Model file for the job. Use its own axes, mm. A direction names the side the tool comes from. Give positions to 0.01 mm unless a question says otherwise; leave off trailing zeros.
```python
from build123d import *

# Parameters (mm, degrees)
SKETCH1_R           = 3.5
BOSS_EXTRUDE1_DEPTH = 3.25
CUT_EXTRUDE1_DEPTH  = 2.75
SKETCH3_R           = 1.5
CUT_EXTRUDE2_DEPTH  = 6.662375826
BOSS_EXTRUDE6_DEPTH = 0.5
BOSS_EXTRUDE4_START = -2
SKETCH6_W           = 3.5
SKETCH6_H           = 2.5
BOSS_EXTRUDE4_DEPTH = 2.5
SKETCH7_W           = 2
SKETCH7_H           = 1.25
CUT_EXTRUDE3_DEPTH  = 2.23
SKETCH8_R           = 0.59
CUT_EXTRUDE4_DEPTH  = 4
CHAMFER3_SIZE       = 0.5
CIRPATTERN1_COUNT   = 3
CHAMFER4_SIZE       = 0.25


# Some blends are built 0.0001 mm under size
with BuildPart() as part:
    # Sketch1 → Boss-Extrude1 (new body)
    with BuildSketch(Plane(origin=(0, 0, 0), x_dir=(1, 0, 0), z_dir=(0, 1, 0))):
        with Locations(Location((0, 0, 0), (0, 0, 90))):
            Circle(SKETCH1_R)
    extrude(amount=BOSS_EXTRUDE1_DEPTH)

    # Sketch2 → Cut-Extrude1 (cut)
    with BuildSketch(Plane(origin=(0, 3.25, 0), x_dir=(1, 0, 0), z_dir=(0, 1, 0))):
        Polygon((1.327905619, -2.3), (2.655811238, 0), (1.327905619, 2.3), (-1.327905619, 2.3), (-2.655811238, 0), (-1.327905619, -2.3), align=None)
    extrude(amount=-CUT_EXTRUDE1_DEPTH, mode=Mode.SUBTRACT)

    # Sketch3 → Cut-Extrude2 (cut, through all)
    with BuildSketch(Plane(origin=(0, 0.5, 0), x_dir=(1, 0, 0), z_dir=(0, 1, 0))):
        with Locations(Location((0, 0, 0), (0, 0, 270))):
            Circle(SKETCH3_R)
    extrude(amount=-CUT_EXTRUDE2_DEPTH, mode=Mode.SUBTRACT)

    # Sketch4 → Boss-Extrude6 (add)
    with BuildSketch(Plane.XZ):
        with BuildLine():
            Line((-1.5, 4.5), (-1.5, 3.16227766))
            ThreePointArc((-1.5, 3.16227766), (0, 3.5), (1.5, 3.16227766))
            Line((1.5, 3.16227766), (1.5, 4.5))
            Line((1.5, 4.5), (1.5, 6))
            Line((1.5, 6), (-1.5, 6))
            Line((-1.5, 6), (-1.5, 4.5))
        make_face()
        with BuildLine():
            Line((4.647114317, -0.950961894), (3.488612788, -0.282100724))
            ThreePointArc((3.488612788, -0.282100724), (3.031088913, -1.75), (1.988612788, -2.880176936))
            Line((1.988612788, -2.880176936), (3.147114317, -3.549038106))
            Line((3.147114317, -3.549038106), (4.647114317, -0.950961894))
        make_face()
        with BuildLine():
            Line((-3.147114317, -3.549038106), (-1.988612788, -2.880176936))
            ThreePointArc((-1.988612788, -2.880176936), (-3.031088913, -1.75), (-3.488612788, -0.282100724))
            Line((-3.488612788, -0.282100724), (-4.647114317, -0.950961894))
            Line((-4.647114317, -0.950961894), (-3.147114317, -3.549038106))
        make_face()
        with BuildLine():
            Line((1.5, -4.5), (1.5, -3.16227766))
            ThreePointArc((1.5, -3.16227766), (0, -3.5), (-1.5, -3.16227766))
            Line((-1.5, -3.16227766), (-1.5, -4.5))
            Line((-1.5, -4.5), (-1.5, -6))
            Line((-1.5, -6), (1.5, -6))
            Line((1.5, -6), (1.5, -4.5))
        make_face()
    extrude(amount=-BOSS_EXTRUDE6_DEPTH)

    # Sketch6 → Boss-Extrude4 (add)
    with BuildSketch(Plane.XY.offset(-2.8).offset(BOSS_EXTRUDE4_START)):
        with Locations((0, 2)):
            Rectangle(SKETCH6_W, SKETCH6_H)
    boss_extrude4 = extrude(amount=BOSS_EXTRUDE4_DEPTH)

    # Sketch7 → Cut-Extrude3 (cut)
    with BuildSketch(Plane(origin=(0, 3.25, 0), x_dir=(1, 0, 0), z_dir=(0, 1, 0))):
        with Locations((0, 3.425)):
            Rectangle(SKETCH7_W, SKETCH7_H)
    cut_extrude3 = extrude(amount=-CUT_EXTRUDE3_DEPTH, mode=Mode.SUBTRACT)

    # Sketch8 → Cut-Extrude4 (cut)
    with BuildSketch(Plane(origin=(0, 0, -4.8), x_dir=(-1, 0, 0), z_dir=(0, 0, -1))):
        with Locations((0, 2.2)):
            Circle(SKETCH8_R)
    cut_extrude4 = extrude(amount=-CUT_EXTRUDE4_DEPTH, mode=Mode.SUBTRACT)

    # Chamfer3
    # the kernel refuses this chamfer: 0.5 mm, written as the material it takes off along each edge
    with BuildSketch(Plane(origin=(0, 0, 0), x_dir=(-0.90124662040542, 0, -0.4333065072299383), z_dir=(0.4333065072299383, 0, -0.90124662040542))) as chamfer3_piece_1_section:
        Polygon((3.5, CHAMFER3_SIZE), (3.5 - CHAMFER3_SIZE, 0), (3.5, 0), align=None)
    chamfer3_piece_1 = revolve(axis=Axis((0, 0, 0), (0, 1, 0)), revolution_arc=111.355166333, mode=Mode.PRIVATE)
    chamfer3_piece_1 = split(chamfer3_piece_1, bisect_by=Plane(origin=(-2.813419939, 0.5, 1.624328759), z_dir=(0, -1, 0)), keep=Keep.TOP, mode=Mode.PRIVATE)
    chamfer3_piece_1 = split(chamfer3_piece_1, bisect_by=Plane(origin=(-2.15670997, 0.237200346, 0.486873726), z_dir=(-0.5000000000000004, 0, 0.8660254037844385)), keep=Keep.TOP, mode=Mode.PRIVATE)
    chamfer3_piece_1 = split(chamfer3_piece_1, bisect_by=Plane(origin=(-1.5, 0.237200346, 1.624328759), z_dir=(-1, 0, 0)), keep=Keep.TOP, mode=Mode.PRIVATE)
    add(chamfer3_piece_1, mode=Mode.SUBTRACT)
    with BuildSketch(Plane(origin=(0, 0, 0), x_dir=(0.8258293731996098, 0, -0.5639200708972323), z_dir=(0.5639200708972323, 0, 0.8258293731996098))) as chamfer3_piece_2_section:
        Polygon((3.5, CHAMFER3_SIZE), (3.5 - CHAMFER3_SIZE, 0), (3.5, 0), align=None)
    chamfer3_piece_2 = revolve(axis=Axis((0, 0, 0), (0, 1, 0)), revolution_arc=51.345334665, mode=Mode.PRIVATE)
    chamfer3_piece_2 = split(chamfer3_piece_2, bisect_by=Plane(origin=(1.689638758, 0.5, -2.926540175), z_dir=(0, -1, 0)), keep=Keep.TOP, mode=Mode.PRIVATE)
    chamfer3_piece_2 = split(chamfer3_piece_2, bisect_by=Plane(origin=(1.784458137, 0.189171232, -2.762308193), z_dir=(-0.5000000000000001, 0, -0.8660254037844386)), keep=Keep.TOP, mode=Mode.PRIVATE)
    chamfer3_piece_2 = split(chamfer3_piece_2, bisect_by=Plane(origin=(1.5, 0.189171232, -2.926540175), z_dir=(1, 0, 0)), keep=Keep.TOP, mode=Mode.PRIVATE)
    add(chamfer3_piece_2, mode=Mode.SUBTRACT)
    with BuildSketch(Plane(origin=(0, 0, 0), x_dir=(0.0753688673164782, 0, 0.9971557219609338), z_dir=(-0.9971557219609338, 0, 0.0753688673164782))) as chamfer3_piece_3_section:
        Polygon((3.5, CHAMFER3_SIZE), (3.5 - CHAMFER3_SIZE, 0), (3.5, 0), align=None)
    chamfer3_piece_3 = revolve(axis=Axis((0, 0, 0), (0, 1, 0)), revolution_arc=111.355166333, mode=Mode.PRIVATE)
    chamfer3_piece_3 = split(chamfer3_piece_3, bisect_by=Plane(origin=(2.813419939, 0.5, 1.624328759), z_dir=(0, -1, 0)), keep=Keep.TOP, mode=Mode.PRIVATE)
    chamfer3_piece_3 = split(chamfer3_piece_3, bisect_by=Plane(origin=(1.5, 0.237200346, 1.624328759), z_dir=(1, 0, 0)), keep=Keep.TOP, mode=Mode.PRIVATE)
    chamfer3_piece_3 = split(chamfer3_piece_3, bisect_by=Plane(origin=(2.15670997, 0.237200346, 0.486873726), z_dir=(0.4999999999999997, 0, 0.8660254037844388)), keep=Keep.TOP, mode=Mode.PRIVATE)
    add(chamfer3_piece_3, mode=Mode.SUBTRACT)

    # CirPattern1: Boss-Extrude4, Cut-Extrude3, Cut-Extrude4 ×3 about axis
    cirpattern1_axis = Axis((0, 0, 0), (0, 1, 0))
    add([boss_extrude4.rotate(cirpattern1_axis, i * 360 / CIRPATTERN1_COUNT) for i in range(1, CIRPATTERN1_COUNT)])
    add([cut_extrude3.rotate(cirpattern1_axis, i * 360 / CIRPATTERN1_COUNT) for i in range(1, CIRPATTERN1_COUNT)], mode=Mode.SUBTRACT)
    add([cut_extrude4.rotate(cirpattern1_axis, i * 360 / CIRPATTERN1_COUNT) for i in range(1, CIRPATTERN1_COUNT)], mode=Mode.SUBTRACT)

    # Chamfer4
    chamfer4_edges = [part.edges().sort_by_distance(p)[0] for p in [
        (0, 0, -1.5),
        (0, 0.5, -1.5),
    ]]
    chamfer(chamfer4_edges, length=CHAMFER4_SIZE - 0.0001)  # a hair under: the kernel refuses the full size


solid = part.part
```
1. Pin check, flat tips, straight feed: P1, Ø1.8, axis at x = 0, z = 0, coming from the +Y side; P2, Ø1.6, axis at x = 2.5, z = 3, coming from the -Y side; P3, Ø0.9, axis at x = 0, z = 4, coming from the +Y side; P4, Ø1.6, axis at x = -0.5, y = 2.5, coming from the +Z side. Stop position of each tip, or through.
Calculated:
P1: passes through
P2: stops at y = 0.11
P3: stops at y = 0.5
P4: stops at z = 3.5
2. Slice it at A-A, the plane x = 0. State how many separate pieces and enclosed holes the cut face has, and give its area (3 significant figures).
Calculated:
separate pieces: 4
enclosed holes: 0
area: 9.96 mm2
3. Pull direction Z, two halves, no side cores. Call faces 1 (the flat face through (-2.001, 1.283, 1.134)), 2 (the flat face through (-2.53, 1.98, 3.48)), 3 (the flat face through (1.75, 2, -4)): +Z half, -Z half, draft (parallel to the pull), parting line (faces both ways), or undercut.
Calculated:
face 1: undercut
face 2: +Z half
face 3: draft
4. Which spindle directions (+Z, -Z, +X, -X, +Y, -Y) get a long thin tool onto all of the face, cutting with end or side? Do faces 4 (the cylindrical face through (0.128, 1.624, -4.43)), 5 (the flat face through (-1.75, 2, -4)), 6 (the flat face through (0, 3, -4.05)). Say none if no direction does.
Calculated:
face 4: -Z
face 5: -Z, -X, +Y, -Y
face 6: +Y
5. Probe probe 1 along Y at (x, z) = (0, -4.45); probe 2 along Y at (x, z) = (0, -2.55); probe 3 along Z at (x, y) = (2.5, 1.25). List the from-to ranges inside material, lowest first.
Calculated:
probe 1: y = 0 to 0.5, 0.75 to 1.61, 2.79 to 3.25
probe 2: y = 0 to 1.61, 2.79 to 3.25
probe 3: z = -2.45 to -0.27, 0.27 to 1.27, 2.6 to 3.46
